Could you check a few things on this model? Use its own coordinates, in mm. Coordinates: 2 decimals unless noted, no trailing zeros. Loops run counter-clockwise (first coordinate to the right, second up) from the corner with the lowest first, then second, coordinate; pieces in that order, holes last. Notation, with made-up numbers: (49, 84.25) - (55, 84.25) arc R16 ccw to (55, 88.25) - close; hole circle Ø3 at (41.25, 17). An arc over 180 degrees is marked (long way). Put each result on its own line as item: value. Start each with the question number.
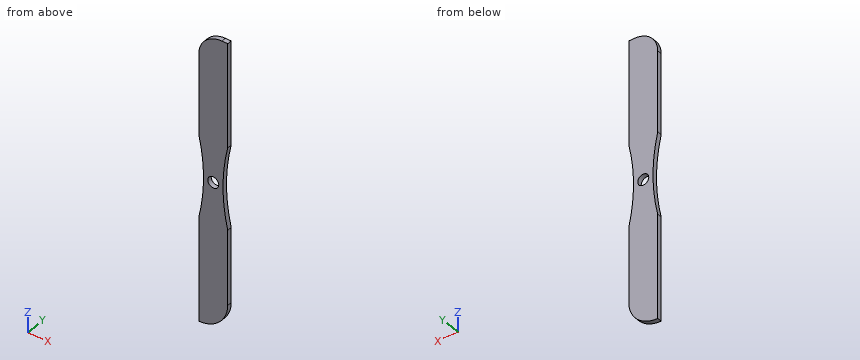
```python
from build123d import *

# Parameters (mm, degrees)
F0_R     = 2.413
F1_DEPTH = 2


with BuildPart() as f1:
    # F0 (on Front) → F1 (new body)
    with BuildSketch(Plane.XZ):
        with BuildLine():
            Line((6.35, 63.5), (3.81, 63.5))
            ThreePointArc((3.81, 63.5), (-3.374205, 60.524205), (-6.35, 53.34))
            Line((-6.35, 53.34), (-6.35, 18.002914))
            ThreePointArc((-6.35, 18.002914), (-4.280137, 0), (-6.35, -18.002914))
            Line((-6.35, -18.002914), (-6.35, -63.5))
            ThreePointArc((-6.35, -63.5), (2.630256, -59.780256), (6.35, -50.8))
            Line((6.35, -50.8), (6.35, -18.002914))
            ThreePointArc((6.35, -18.002914), (4.278073, 0), (6.35, 18.002914))
            Line((6.35, 18.002914), (6.35, 63.5))
        make_face()
        Circle(F0_R, mode=Mode.SUBTRACT)
    extrude(amount=F1_DEPTH)


solid = f1.part
```
(1) For pin 1 Ø3 at (x, z) = (0, 0) entering from +Y, with a flat end and sliding along its axis, tell me the tip position at first contact or that it passes through.
(2) I want a section at D-D on z = 16.5. List the corners of the cut face in (x, y) for me.
(3) I want a section at C-C on x = -0.25. List the corners of the cut face in (y, z) for me, and give its area (3 significant figures).
(4) I want a section at A-A on y = -1.6. List the corners of the cut face in (x, z) for me, and give its area (3 significant figures).
(5) I need wall thicknesses on L1, parallel to Z at x = 0.5, y = -1.7; L2, parallel to Z at x = 0, y = -0.35; L3, parallel to Z at x = -4.25, y = -0.7. Which ranges of each line are inside material? Lowest first, please. Write a range as [from, to].
(6) I want a section at B-B on z = 0. List the corners of the cut face in (x, y) for me.
Answer sheet:
1. pin 1: passes through
2. outline: (-6.02, -2) - (6.01, -2) - (6.01, 0) - (-6.02, 0) - close
3. outline: (-2, -61.94) - (0, -61.94) - (0, -2.4) - (-2, -2.4) - close; (-2, 2.4) - (0, 2.4) - (0, 62.65) - (-2, 62.65) - close
3. area: 240 mm^2
4. outline: (-6.35, -63.5) arc R12.7 ccw to (6.35, -50.8) - (6.35, -18) arc R79.25 cw to (6.35, 18) - (6.35, 63.5) - (3.81, 63.5) arc R10.16 ccw to (-6.35, 53.34) - (-6.35, 18) arc R79.33 cw to (-6.35, -18) - close; hole circle Ø4.83 at (0, 0)
4. area: 1,440 mm^2
5. L1: z = [-61.49, -2.36], [2.36, 62.95]
5. L2: z = [-61.8, -2.41], [2.41, 62.76]
5. L3: z = [-63.33, 59.53]
6. outline: (-4.28, -2) - (-2.41, -2) - (-2.41, 0) - (-4.28, 0) - close; (2.41, -2) - (4.28, -2) - (4.28, 0) - (2.41, 0) - close
